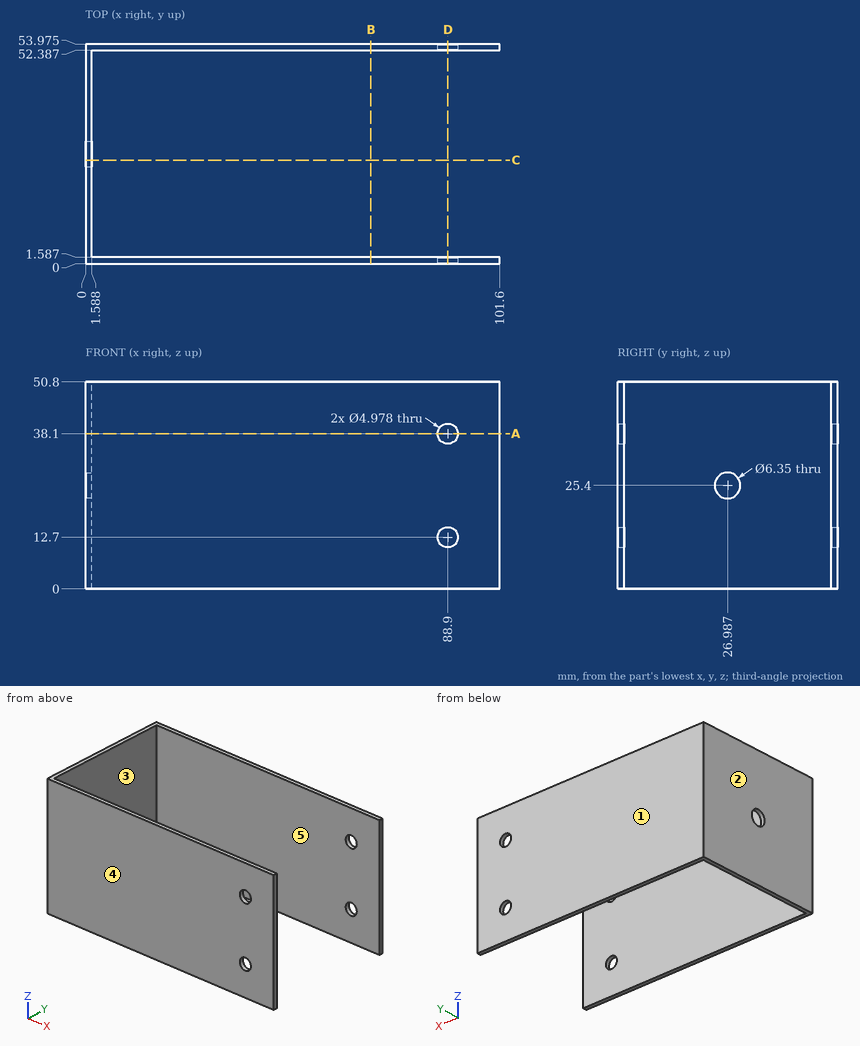
Geometry check sheet. Reference: drawing and pictorial views, mm from the part's lowest x, y, z. A direction names the side the tool comes from. Round coordinates to 2 decimals unless told otherwise and drop trailing zeros. Loops run counter-clockwise (first coordinate to the right, second up) from the corner with the lowest first, then second, coordinate; pieces in that order, holes last. Notation, with made-up numbers: (-33, 18) - (-27, 18) arc R27 ccw to (-27, 47) - close; hole circle Ø7 at (-37.5, -33). An arc over 180 degrees is marked (long way). Answer as CSV lines item,"result".
(1) Material ranges on line 1 along Z through (x, y) = (88.9, 1.2); line 2 along Y through (x, z) = (42.5, 41.5) (1 decimal); line 3 along X through (y, z) = (0.95, 12.7), recorded low to high.
Output values:
line 1,"z = 0 to 10.21, 15.19 to 35.61, 40.59 to 50.8"
line 2,"y = 0 to 1.6, 52.4 to 54"
line 3,"x = 0 to 86.41, 91.39 to 101.6"
(2) Depth check by flat-ended pin: pin 1 Ø1 at (y, z) = (8, 36.5) entering from +X; pin 2 Ø4.5 at (x, z) = (88.9, 12.7) entering from +Y. Enter the tip coordinate at first touch or a pass-through.
Output values:
pin 1,"stops at x = 1.59"
pin 2,"passes through"
(3) Cross-section at C-C, the plane y = 25.5. Enter the section's corners in (x, z) (1 decimal).
Output values:
outline,"(0, 0) - (1.6, 0) - (1.6, 22.6) - (0, 22.6) - close; (0, 28.2) - (1.6, 28.2) - (1.6, 50.8) - (0, 50.8) - close"
(4) Cross-section at A-A, the plane z = 38.1. Enter the section's corners in (x, y) (1 decimal).
Output values:
outline,"(0, 0) - (86.4, 0) - (86.4, 1.6) - (1.6, 1.6) - (1.6, 52.4) - (86.4, 52.4) - (86.4, 54) - (0, 54) - close; (91.4, 0) - (101.6, 0) - (101.6, 1.6) - (91.4, 1.6) - close; (91.4, 52.4) - (101.6, 52.4) - (101.6, 54) - (91.4, 54) - close"
(5) Cross-section at D-D, the plane x = 88.9. Enter the section's corners in (y, z) (1 decimal).
Output values:
outline,"(0, 0) - (1.6, 0) - (1.6, 10.2) - (0, 10.2) - close; (0, 15.2) - (1.6, 15.2) - (1.6, 35.6) - (0, 35.6) - close; (0, 40.6) - (1.6, 40.6) - (1.6, 50.8) - (0, 50.8) - close; (52.4, 0) - (54, 0) - (54, 10.2) - (52.4, 10.2) - close; (52.4, 15.2) - (54, 15.2) - (54, 35.6) - (52.4, 35.6) - close; (52.4, 40.6) - (54, 40.6) - (54, 50.8) - (52.4, 50.8) - close"
(6) Release check for a two-part mould opening along Y. For the marked faces 1, 2 and 3 record: released by +Y, released by -Y, zero draft, split by the parting line, or undercut.
Output values:
face 1,"released by +Y"
face 2,"zero draft"
face 3,"undercut"
(7) Cross-section at B-B, the plane x = 70. Enter the section's corners in (y, z) (1 decimal).
Output values:
outline,"(0, 0) - (1.6, 0) - (1.6, 50.8) - (0, 50.8) - close; (52.4, 0) - (54, 0) - (54, 50.8) - (52.4, 50.8) - close"
(8) Set-up check for the marked faces 4 and 5: record each of +Z, -Z, +X, -X, +Y, -Y from which the full face is reachable in a straight line by a thin tool's end or side.
Output values:
face 4,"+Z, -Z, +X, -X, -Y"
face 5,"+Z, -Z, +X"
